Model file for the job. Use its own axes, mm. Round coordinates to 2 decimals unless told otherwise and drop trailing zeros. Order: outer loops, then holes, each group sorted by start corner. A loop starts at its lowest first (then second) coordinate and runs counter-clockwise, first axis right, second up. Notation, with made-up numbers: (80.25, -19.5) -> (102.25, -19.5) arc R27 ccw to (102.25, 6.5) -> close; hole circle Ø2 at (-12, 32). An arc over 180 degrees is marked (long way). Put each result on its own line as item: value. Start each with the question number.
Q1. Flat gauge pins, fed straight in: P1, Ø12, axis at x = 46.5, y = 242.5, coming from the -Z side; P2, Ø2, axis at x = 2.5, z = 1, coming from the +Y side. Where does each tip first touch, or does it go through?
Q2. Cut at B-B, the plane y = 210.5. List the corners of the cut face in (x, z).
Q3. Probe L1, parallel to X at y = 214, z = 3.4; L2, parallel to Y at x = 44, z = 2.85; L3, parallel to Y at x = 3.5, z = 0.45. List the from-to ranges inside material, lowest first.
Q4. Cut at A-A, the plane z = 1.6. List the corners of the cut face in (x, y), and give its area (3 significant figures).
from build123d import *

# Parameters (mm, degrees)
BOSS_EXTRUDE1_DEPTH = 4
SKETCH2_W           = 4
SKETCH2_H           = 92
CUT_EXTRUDE1_DEPTH  = 309.784714648


with BuildPart() as part:
    # Sketch1 → Boss-Extrude1 (new body)
    with BuildSketch(Plane.XY):
        Polygon((0, 300), (4, 300), (4, 304), (50, 304), (50, 300), (54, 300), (54, 0), (0, 0), align=None)
    extrude(amount=BOSS_EXTRUDE1_DEPTH)

    # Sketch2 → Cut-Extrude1 (cut, through all)
    with BuildSketch(Plane.XY.offset(4)):
        with Locations((44, 198)):
            Rectangle(SKETCH2_W, SKETCH2_H)
    extrude(amount=-CUT_EXTRUDE1_DEPTH, mode=Mode.SUBTRACT)


solid = part.part
Ans:
1. P1: stops at z = 0
1. P2: stops at y = 300
2. outline: (0, 0) -> (42, 0) -> (42, 4) -> (0, 4) -> close; (46, 0) -> (54, 0) -> (54, 4) -> (46, 4) -> close
3. L1: x = 0 to 42, 46 to 54
3. L2: y = 0 to 152, 244 to 304
3. L3: y = 0 to 300
4. outline: (0, 0) -> (54, 0) -> (54, 300) -> (50, 300) -> (50, 304) -> (4, 304) -> (4, 300) -> (0, 300) -> close; hole (42, 152) -> (46, 152) -> (46, 244) -> (42, 244) -> close
4. area: 16,000 mm^2
